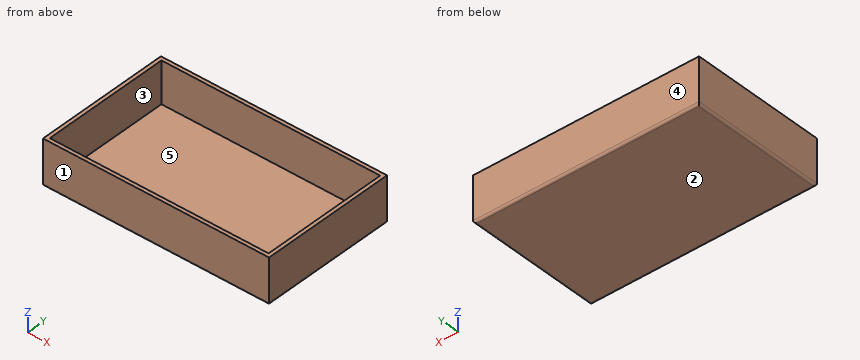
from build123d import *

# Parameters (mm, degrees)
F0_W     = 100
F0_H     = 60
F1_DEPTH = 20
F2_T     = -1.6
F3_R     = 1


with BuildPart() as f1:
    # F0 (on Top) → F1 (new body)
    with BuildSketch(Plane.XY):
        with Locations((-19.466264, 3.285318)):
            Rectangle(F0_W, F0_H)
    extrude(amount=F1_DEPTH)

    # F2
    f2_openings = [f1.faces().sort_by_distance(p)[0] for p in [
        (-19.466264, 3.285318, 20),
    ]]
    offset(amount=F2_T, openings=f2_openings)

    # F3
    f3_edges = [f1.edges().sort_by_distance(p)[0] for p in [
        (-69.466264, 3.285318, 0),
        (-19.466264, -26.714682, 0),
        (30.533736, 3.285318, 0),
        (-19.466264, 33.285318, 0),
    ]]
    fillet(f3_edges, radius=F3_R)


solid = f1.part
Verification items for the finished model (mm, model axes). Face numbers are marked on the shaded views. A direction names the side the tool comes from. Coordinates: 2 decimals unless noted, no trailing zeros. Loops run counter-clockwise (first coordinate to the right, second up) from the corner with the lowest first, then second, coordinate; pieces in that order, holes last. Notation, with made-up numbers: (-16, 4) -> (43, 4) arc R11 cw to (43, 11) -> close; hole circle Ø1 at (76.5, 7). An arc over 180 degrees is marked (long way). Answer as a JSON object with one key per item and string values. Group by question number.
Item 1: Scan lines: probe 1 along X at (y, z) = (22.5, 16); probe 2 along Y at (x, z) = (-40, 7); probe 3 along Z at (x, y) = (-25.5, -7). Record each from-to range of solid material in increasing order.
Item 2: Depth check by flat-ended pin: pin 1 (1.5 mm diameter, centred on x = -28.5, y = 24.5, fed in from +Z). Enter the tip coordinate at first touch or a pass-through.
Item 3: Mould release check, pull along Y, two halves, no side actions. Record for the marked faces 1, 2 and 3: +Y half, -Y half, draft (parallel to the pull), parting line (faces both ways), or undercut.
Item 4: Sectioned sample at A-A on z = 9.5. Record the boundary of the cut face in (x, y), plus the area to 3 significant figures.
Item 5: Sectioned sample at B-B on y = -19.5. Record the boundary of the cut face in (x, z).
Item 6: Sectioned sample at C-C on x = -2. Record the boundary of the cut face in (y, z).
Item 7: Tool access check on the marked faces 4 and 5. Record the directions out of +Z, -Z, +X, -X, +Y, -Y that give a thin tool (end or side, any length) a straight path to the whole face; none if there is none.
Evaluation:
{
 "1": {"probe 1": "x = -69.47 to -67.87, 28.93 to 30.53", "probe 2": "y = -26.71 to -25.11, 31.69 to 33.29", "probe 3": "z = 0 to 1.6"},
 "2": {"pin 1": "stops at z = 1.6"},
 "3": {"face 1": "-Y half", "face 2": "draft", "face 3": "undercut"},
 "4": {"outline": "(-69.47, -26.71) -> (30.53, -26.71) -> (30.53, 33.29) -> (-69.47, 33.29) -> close; hole (-67.87, -25.11) -> (28.93, -25.11) -> (28.93, 31.69) -> (-67.87, 31.69) -> close", "area": "502 mm²"},
 "5": {"outline": "(-69.47, 1) arc R1 ccw to (-68.47, 0) -> (29.53, 0) arc R1 ccw to (30.53, 1) -> (30.53, 20) -> (28.93, 20) -> (28.93, 1.6) -> (-67.87, 1.6) -> (-67.87, 20) -> (-69.47, 20) -> close"},
 "6": {"outline": "(-26.71, 1) arc R1 ccw to (-25.71, 0) -> (32.29, 0) arc R1 ccw to (33.29, 1) -> (33.29, 20) -> (31.69, 20) -> (31.69, 1.6) -> (-25.11, 1.6) -> (-25.11, 20) -> (-26.71, 20) -> close"},
 "7": {"face 4": "+Z, -Z, +X, -X, +Y", "face 5": "+Z"}
}
